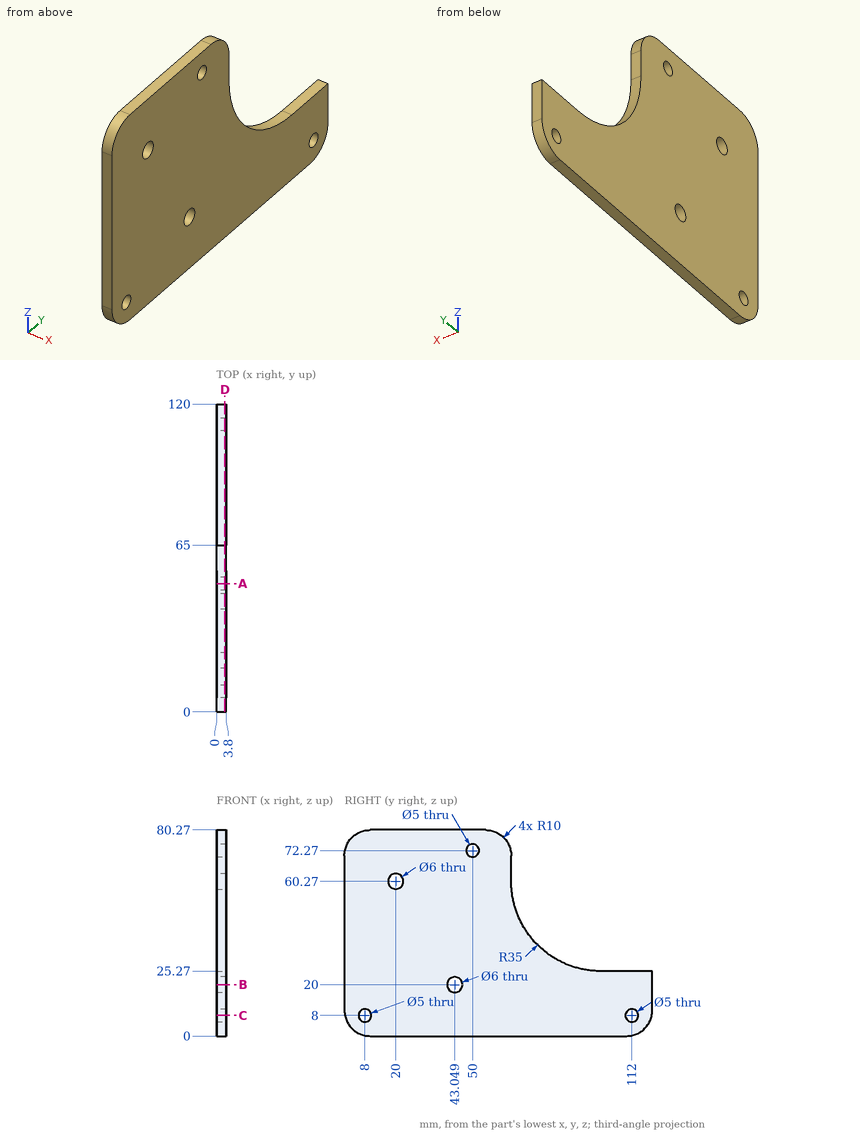
The figure shows three views and two pictorial views of one solid part (mm, origin at its lowest corner). Answer the questions. Round coordinates to 2 decimals unless told otherwise and drop trailing zeros. Order: outer loops, then holes, each group sorted by start corner. A loop starts at its lowest first (then second) coordinate and runs counter-clockwise, first axis right, second up. Notation, with made-up numbers: (51, 8) -> (104, 8) arc R19 cw to (104, 16) -> close; hole circle Ø4 at (-32, -10.5). An arc over 180 degrees is marked (long way). Put each result on its own line as item: value.
Q1. Consider line 1 along Y through (x, z) = (2.95, 8); line 2 along Y through (x, z) = (1.6, 20); line 3 along Y through (x, z) = (3.45, 63.5). Determine where each line is inside the solid, lowest interval first.
Results list:
line 1: 0.2 to 5.5, 10.5 to 109.5, 114.5 to 119.8
line 2: 0 to 40.05, 46.05 to 120
line 3: 0 to 65
Q2. Section C-C, the plane z = 8 is taken. Write down the section's boundary in (x, y).
Results list:
outline: (0, 0.2) -> (3.8, 0.2) -> (3.8, 5.5) -> (0, 5.5) -> close; (0, 10.5) -> (3.8, 10.5) -> (3.8, 109.5) -> (0, 109.5) -> close; (0, 114.5) -> (3.8, 114.5) -> (3.8, 119.8) -> (0, 119.8) -> close
Q3. Section B-B, the plane z = 20 is taken. Write down the section's boundary in (x, y), and give its area (3 significant figures).
Results list:
outline: (0, 0) -> (3.8, 0) -> (3.8, 40.05) -> (0, 40.05) -> close; (0, 46.05) -> (3.8, 46.05) -> (3.8, 120) -> (0, 120) -> close
area: 433 mm^2
Q4. Each of these flat-tipped pins is pushed along its axis until it touches: P1, Ø1.5, axis at x = 1, z = 34.5, coming from the -Y side; P2, Ø2, axis at x = 1.5, z = 40, coming from the +Y side (1 decimal). Where does it stop, or does it pass through?
Results list:
P1: y = 0
P2: y = 72.2
Q5. Section D-D, the plane x = 3.2 is taken. Write down the section's boundary in (y, z), and give its area (3 significant figures).
Results list:
outline: (0, 10) arc R10 ccw to (10, 0) -> (110, 0) arc R10 ccw to (120, 10) -> (120, 25.27) -> (100, 25.27) arc R35 cw to (65, 60.27) -> (65, 70.27) arc R10 ccw to (55, 80.27) -> (10, 80.27) arc R10 ccw to (0, 70.27) -> close; hole circle Ø5 at (8, 8); hole circle Ø6 at (20, 60.27); hole circle Ø6 at (43.05, 20); hole circle Ø5 at (50, 72.27); hole circle Ø5 at (112, 8)
area: 6,670 mm^2
Q6. Section A-A, the plane y = 50 is taken. Write down the section's boundary in (x, z), and give its area (3 significant figures).
Results list:
outline: (0, 0) -> (3.8, 0) -> (3.8, 69.77) -> (0, 69.77) -> close; (0, 74.77) -> (3.8, 74.77) -> (3.8, 80.27) -> (0, 80.27) -> close
area: 286 mm^2
